Verification items for the finished model (mm, model axes). Give positions to 0.01 mm unless a question says otherwise; leave off trailing zeros. Write each loop counter-clockwise with the first axis right and the second up, starting at its lowest first coordinate (ties: lowest second). Pieces come first, ordered by that corner, then holes.
from build123d import *

# Parameters (mm, degrees)
CYLINDER043_R     = 1.5
CYLINDER043_DEPTH = 10
CYLINDER044_R     = 1.5
CYLINDER044_DEPTH = 10
CYLINDER042_R     = 1.5
CYLINDER042_DEPTH = 10
BOX020_W          = 58
BOX020_H          = 10
BOX020_DEPTH      = 10
FILLET009_R       = 3


with BuildPart() as cylinder043:
    # Cylinder043 → Cylinder043 (new body)
    with BuildSketch(Plane(origin=(28, 11, 14), x_dir=(1, 0, 0), z_dir=(0, -1, 0))):
        Circle(CYLINDER043_R)
    extrude(amount=CYLINDER043_DEPTH)


with BuildPart() as cylinder044:
    # Cylinder044 → Cylinder044 (new body)
    with BuildSketch(Plane(origin=(51, 11, 14), x_dir=(1, 0, 0), z_dir=(0, -1, 0))):
        Circle(CYLINDER044_R)
    extrude(amount=CYLINDER044_DEPTH)


with BuildPart() as fusion033:
    # Cylinder042 → Cylinder042 (new body)
    with BuildSketch(Plane(origin=(6, 11, 14), x_dir=(1, 0, 0), z_dir=(0, -1, 0))):
        Circle(CYLINDER042_R)
    extrude(amount=CYLINDER042_DEPTH)

    # Fusion033: union Cylinder043, Cylinder044
    add(cylinder043.part)
    add(cylinder044.part)


with BuildPart() as frame_holes001:
    # Box020 → Box020 (new body)
    with BuildSketch(Plane.XY.offset(9)):
        with Locations((29, 5)):
            Rectangle(BOX020_W, BOX020_H)
    extrude(amount=BOX020_DEPTH)

    # Fillet009
    fillet009_edges = [frame_holes001.edges().sort_by_distance(p)[0] for p in [
        (29, 0, 19),
    ]]
    fillet(fillet009_edges, radius=FILLET009_R)


with BuildPart() as frame_holes001_1:
    # Fillet009 placement: moved
    add(frame_holes001.part.moved(Location((-0.5, 1, 0))))

    # Cut018: cut Fusion033
    add(fusion033.part, mode=Mode.SUBTRACT)


solid = frame_holes001_1.part
Item 1: Sectioned sample at B-B on z = 14. Record the cut outline in (x, y).
Answer key:
outline: (-0.5, 1) - (4.5, 1) - (4.5, 11) - (-0.5, 11) - close; (7.5, 1) - (26.5, 1) - (26.5, 11) - (7.5, 11) - close; (29.5, 1) - (49.5, 1) - (49.5, 11) - (29.5, 11) - close; (52.5, 1) - (57.5, 1) - (57.5, 11) - (52.5, 11) - close
Item 2: Sectioned sample at D-D on x = 47.5. Record the cut outline in (y, z), then the cut area to 3 significant figures.
Answer key:
outline: (1, 9) - (11, 9) - (11, 19) - (4, 19) arc R3 ccw to (1, 16) - close
area: 98.1 mm2
Item 3: Sectioned sample at A-A on x = 28. Record the cut outline in (y, z), then the cut area to 3 significant figures.
Answer key:
outline: (1, 9) - (11, 9) - (11, 12.5) - (1, 12.5) - close; (1, 15.5) - (11, 15.5) - (11, 19) - (4, 19) arc R3 ccw to (1, 16) - close
area: 68.1 mm2
Item 4: Release check for a two-part mould opening along X. For faces 1 (the face through (28, 11, 16)), 2 (the face through (49.5, 6.07, 14.07)), 3 (the face through (57.5, 6, 14)) record: released by +X, released by -X, zero draft, split by the parting line, or undercut.
Answer key:
face 1: zero draft
face 2: undercut
face 3: released by +X
Item 5: Scan lines: line 1 along Z through (x, y) = (51, 6.25); line 2 along X through (y, z) = (10, 14.5); line 3 along Y through (x, z) = (13, 17.5). Record each from-to range of solid material in increasing order.
Answer key:
line 1: z = 9 to 12.5, 15.5 to 19
line 2: x = -0.5 to 4.59, 7.41 to 26.59, 29.41 to 49.59, 52.41 to 57.5
line 3: y = 1.4 to 11
Item 6: Sectioned sample at C-C on y = 7.75. Record the cut outline in (x, z), then the cut area to 3 significant figures.
Answer key:
outline: (-0.5, 9) - (57.5, 9) - (57.5, 19) - (-0.5, 19) - close; hole circle Ø3 at (6, 14); hole circle Ø3 at (28, 14); hole circle Ø3 at (51, 14)
area: 559 mm2
